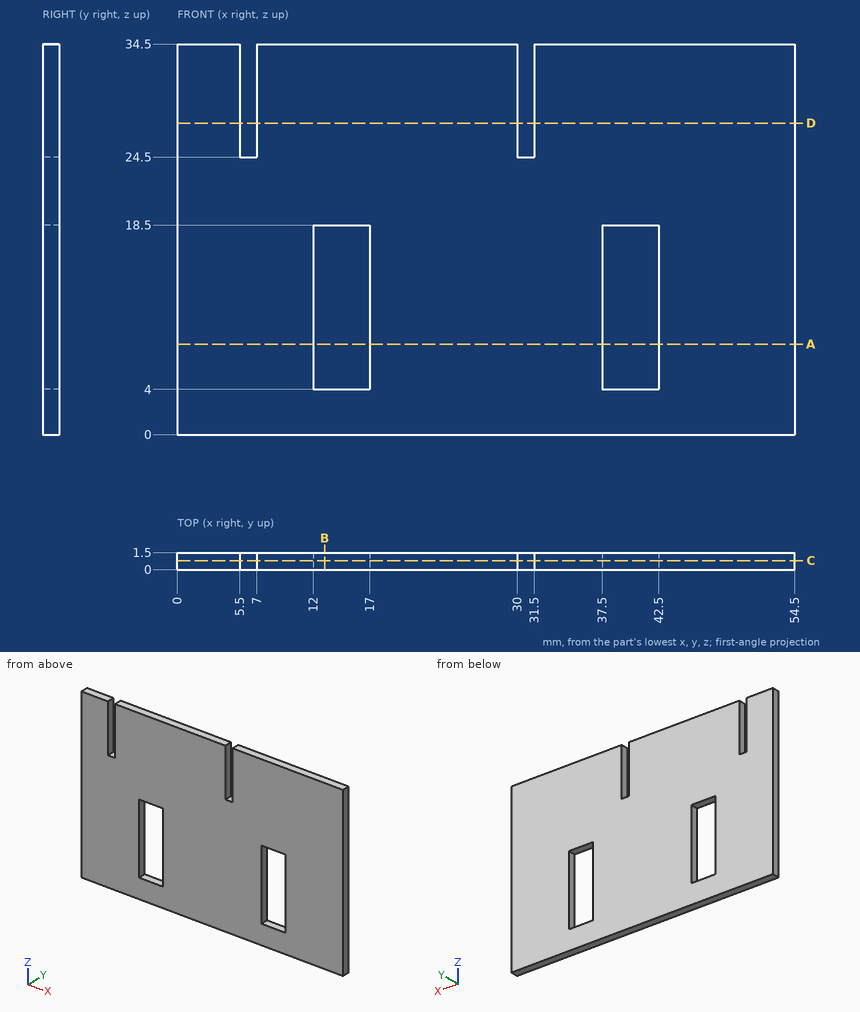
Part print with two shaded views. Sizes in mm from the minimum x, y, z corner. Coordinates: 2 decimals unless noted, no trailing zeros. Write each loop counter-clockwise with the first axis right and the second up, starting at its lowest first coordinate (ties: lowest second). Pieces come first, ordered by that corner, then holes. Notation, with made-up numbers: (-15.5, 28) - (19.5, 28) arc R17 ccw to (19.5, 52) - close; hole circle Ø5 at (55, 75.25). An arc over 180 degrees is marked (long way). Use a Markdown table: item, result. Add a question column.
Item 1: Drill centre lines: line 1 along X through (y, z) = (0.25, 25); line 2 along X through (y, z) = (1.05, 14); line 3 along Z through (x, y) = (41.5, 0.1). Where is each one in solid material? Low to high.
Item 2: Band-saw the part on A-A, the plane z = 8. Write the cut outline in (x, y).
Item 3: Band-saw the part on D-D, the plane z = 27.5. Write the cut outline in (x, y).
Item 4: Band-saw the part on C-C, the plane y = 0.8. Write the cut outline in (x, z), and give its area (3 significant figures).
Item 5: Band-saw the part on B-B, the plane x = 13. Write the cut outline in (y, z), and give its area (3 significant figures).
A:
| question | item | result |
|---|---|---|
| 1 | line 1 | x = 0 to 5.5, 7 to 30, 31.5 to 54.5 |
| 1 | line 2 | x = 0 to 12, 17 to 37.5, 42.5 to 54.5 |
| 1 | line 3 | z = 0 to 4, 18.5 to 34.5 |
| 2 | outline | (0, 0) - (12, 0) - (12, 1.5) - (0, 1.5) - close; (17, 0) - (37.5, 0) - (37.5, 1.5) - (17, 1.5) - close; (42.5, 0) - (54.5, 0) - (54.5, 1.5) - (42.5, 1.5) - close |
| 3 | outline | (0, 0) - (5.5, 0) - (5.5, 1.5) - (0, 1.5) - close; (7, 0) - (30, 0) - (30, 1.5) - (7, 1.5) - close; (31.5, 0) - (54.5, 0) - (54.5, 1.5) - (31.5, 1.5) - close |
| 4 | outline | (0, 0) - (54.5, 0) - (54.5, 34.5) - (31.5, 34.5) - (31.5, 24.5) - (30, 24.5) - (30, 34.5) - (7, 34.5) - (7, 24.5) - (5.5, 24.5) - (5.5, 34.5) - (0, 34.5) - close; hole (12, 4) - (17, 4) - (17, 18.5) - (12, 18.5) - close; hole (37.5, 4) - (42.5, 4) - (42.5, 18.5) - (37.5, 18.5) - close |
| 4 | area | 1,710 mm² |
| 5 | outline | (0, 0) - (1.5, 0) - (1.5, 4) - (0, 4) - close; (0, 18.5) - (1.5, 18.5) - (1.5, 34.5) - (0, 34.5) - close |
| 5 | area | 30.0 mm² |
